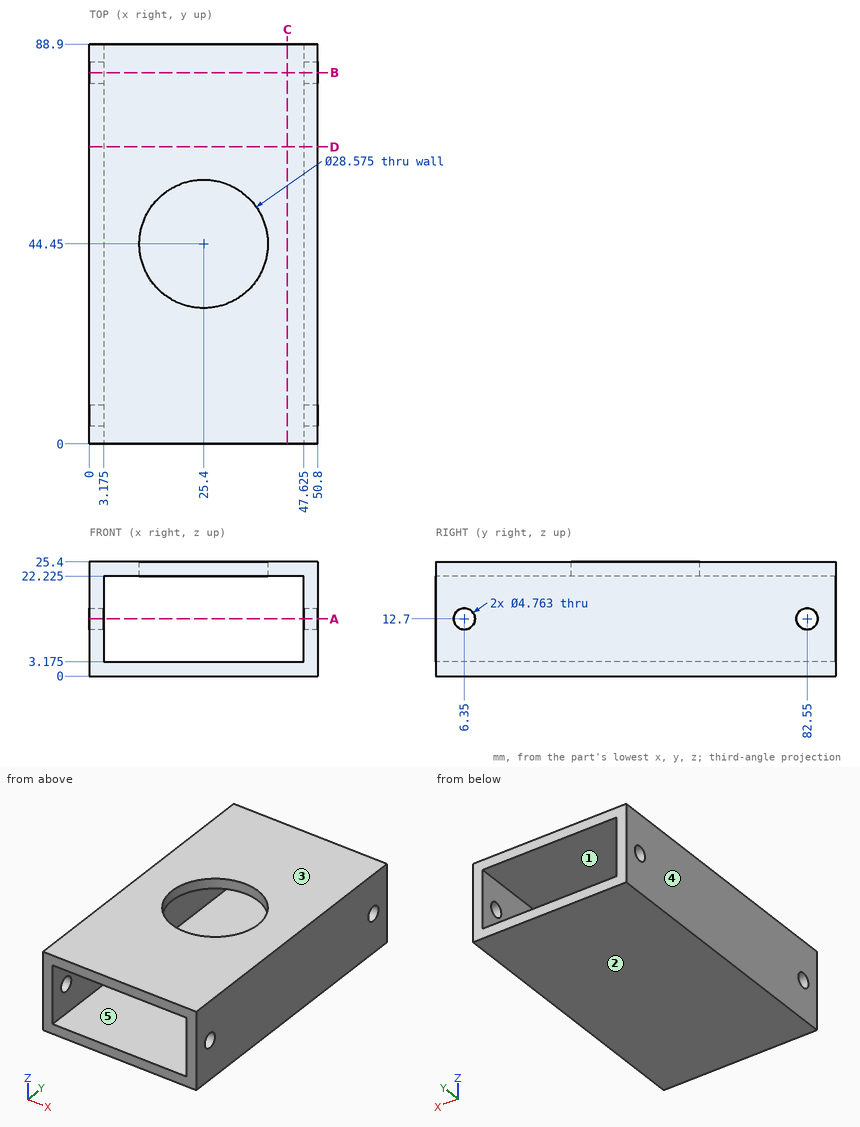
Print and shaded views of the part. All mm, measured from the part's lowest x, y and z. A direction names the side the tool comes from. Coordinates: 2 decimals unless noted, no trailing zeros. Loops run counter-clockwise (first coordinate to the right, second up) from the corner with the lowest first, then second, coordinate; pieces in that order, holes last. Notation, with made-up numbers: (28, 3) -> (78, 3) arc R22 ccw to (78, 37) -> close; hole circle Ø8 at (-6.75, -3). An arc over 180 degrees is marked (long way). Use a Markdown table: item, result. Add a question column.
Item 1: Flat gauge pin, fed straight in: P1, Ø4, axis at y = 6.35, z = 12.7, coming from the +X side. Where does the tip first touch, or does it go through?
Item 2: Pull direction Z, two halves, no side cores. Call the marked faces 1, 2 and 3: +Z half, -Z half, draft (parallel to the pull), parting line (faces both ways), or undercut.
Item 3: Band-saw the part on D-D on y = 66. Write the cut outline in (x, z) (1 decimal).
Item 4: Band-saw the part on A-A on z = 12.7. Write the cut outline in (x, y) (1 decimal), plus the area to 3 significant figures.
Item 5: Band-saw the part on B-B on y = 82.55. Write the cut outline in (x, z) (1 decimal).
Item 6: Probe probe 1 along Y at (x, z) = (2.1, 12.7); probe 2 along X at (y, z) = (44.45, 24.15); probe 3 along Z at (x, y) = (7, 23.5) (1 decimal). List the from-to ranges inside material, lowest first.
Item 7: Which spindle directions (+Z, -Z, +X, -X, +Y, -Y) get a long thin tool onto all of the face, cutting with end or side? Do the marked faces 4 and 5. Say none if no direction does.
Item 8: Band-saw the part on C-C on x = 44. Write the cut outline in (y, z) (1 decimal).
Geometry says:
| question | item | result |
|---|---|---|
| 1 | P1 | through |
| 2 | face 1 | undercut |
| 2 | face 2 | -Z half |
| 2 | face 3 | +Z half |
| 3 | outline | (0, 0) -> (50.8, 0) -> (50.8, 25.4) -> (0, 25.4) -> close; hole (3.2, 3.2) -> (47.6, 3.2) -> (47.6, 22.2) -> (3.2, 22.2) -> close |
| 4 | outline | (0, 0) -> (3.2, 0) -> (3.2, 4) -> (0, 4) -> close; (0, 8.7) -> (3.2, 8.7) -> (3.2, 80.2) -> (0, 80.2) -> close; (0, 84.9) -> (3.2, 84.9) -> (3.2, 88.9) -> (0, 88.9) -> close; (47.6, 0) -> (50.8, 0) -> (50.8, 4) -> (47.6, 4) -> close; (47.6, 8.7) -> (50.8, 8.7) -> (50.8, 80.2) -> (47.6, 80.2) -> close; (47.6, 84.9) -> (50.8, 84.9) -> (50.8, 88.9) -> (47.6, 88.9) -> close |
| 4 | area | 504 mm² |
| 5 | outline | (0, 0) -> (50.8, 0) -> (50.8, 10.3) -> (47.6, 10.3) -> (47.6, 3.2) -> (3.2, 3.2) -> (3.2, 10.3) -> (0, 10.3) -> close; (0, 15.1) -> (3.2, 15.1) -> (3.2, 22.2) -> (47.6, 22.2) -> (47.6, 15.1) -> (50.8, 15.1) -> (50.8, 25.4) -> (0, 25.4) -> close |
| 6 | probe 1 | 0 to 3.97, 8.73 to 80.17, 84.93 to 88.9 |
| 6 | probe 2 | 0 to 11.11, 39.69 to 50.8 |
| 6 | probe 3 | 0 to 3.2, 22.2 to 25.4 |
| 7 | face 4 | +Z, -Z, -X, +Y, -Y |
| 7 | face 5 | +Y, -Y |
| 8 | outline | (0, 0) -> (88.9, 0) -> (88.9, 3.2) -> (0, 3.2) -> close; (0, 22.2) -> (88.9, 22.2) -> (88.9, 25.4) -> (0, 25.4) -> close |
